Source: CAD feature listing. Evaluate the final solid. Frame: model axes, mm. Round coordinates to 2 decimals unless told otherwise and drop trailing zeros. Order: outer loops, then holes, each group sorted by start corner. A loop starts at its lowest first (then second) coordinate and runs counter-clockwise, first axis right, second up. Notation, with made-up numbers: (-28, 67) - (20, 67) arc R4 ccw to (20, 74) - close; hole circle Ø8 at (21, 44.25). An arc over 180 degrees is marked (long way). Put each result on its own line as item: value. Start each with the question number.
1) Section A-A on y = -0.8. Output: boundary loops of the cut face in (x, z), then the cut area to 3 significant figures.
2) Line query: probe 1 along X at (y, z) = (-1.45, -24); probe 2 along X at (y, z) = (-0.6, -25.5); probe 3 along Z at (x, y) = (-55, 0.1). Output: solid intervals per line, ascending. Write a range as [from, to].
3) Contact query for a flat-ended pin moving along its axis: P1, Ø1.3, axis at y = 1, z = 1, coming from the +X side. Output: stop coordinate, or through.
4) Section B-B on z = 11. Output: boundary loops of the cut face in (x, y).
```python
from build123d import *

# Parameters (mm, degrees)
SKETCH1_R           = 2.2479
BOSS_EXTRUDE1_DEPTH = 1.5875


with BuildPart() as part:
    # Sketch1 → Boss-Extrude1 (new, symmetric)
    with BuildSketch(Plane(origin=(0, 0, 0), x_dir=(1, 0, 0), z_dir=(0, 1, 0))):
        with BuildLine():
            Line((-47.25, 6.976491924), (-47.25, -6.976491924))
            ThreePointArc((-47.25, -6.976491924), (-49.69071054, -13.523028631), (-55.821428571, -16.87392511))
            ThreePointArc((-55.821428571, -16.87392511), (-60.419467095, -19.38709747), (-62.25, -24.297))
            ThreePointArc((-62.25, -24.297), (-60.053300859, -29.600300859), (-54.75, -31.797))
            Line((-54.75, -31.797), (54.75, -31.797))
            ThreePointArc((54.75, -31.797), (60.053300859, -29.600300859), (62.25, -24.297))
            ThreePointArc((62.25, -24.297), (60.419467095, -19.38709747), (55.821428571, -16.87392511))
            ThreePointArc((55.821428571, -16.87392511), (49.69071054, -13.523028631), (47.25, -6.976491924))
            Line((47.25, -6.976491924), (47.25, 6.976491924))
            ThreePointArc((47.25, 6.976491924), (49.69071054, 13.523028631), (55.821428571, 16.87392511))
            ThreePointArc((55.821428571, 16.87392511), (60.419467095, 19.38709747), (62.25, 24.297))
            ThreePointArc((62.25, 24.297), (60.053300859, 29.600300859), (54.75, 31.797))
            Line((54.75, 31.797), (-54.75, 31.797))
            ThreePointArc((-54.75, 31.797), (-60.053300859, 29.600300859), (-62.25, 24.297))
            ThreePointArc((-62.25, 24.297), (-60.419467095, 19.38709747), (-55.821428571, 16.87392511))
            ThreePointArc((-55.821428571, 16.87392511), (-49.69071054, 13.523028631), (-47.25, 6.976491924))
        make_face()
        with Locations(Location((54.75, 24.297, 0), (0, 0, 270))):
            Circle(SKETCH1_R, mode=Mode.SUBTRACT)
        with Locations(Location((54.75, -24.297, 0), (0, 0, 270))):
            Circle(SKETCH1_R, mode=Mode.SUBTRACT)
        with Locations(Location((-54.75, -24.297, 0), (0, 0, 270))):
            Circle(SKETCH1_R, mode=Mode.SUBTRACT)
        with Locations(Location((-54.75, 24.297, 0), (0, 0, 270))):
            Circle(SKETCH1_R, mode=Mode.SUBTRACT)
    extrude(amount=BOSS_EXTRUDE1_DEPTH, both=True)


solid = part.part
```
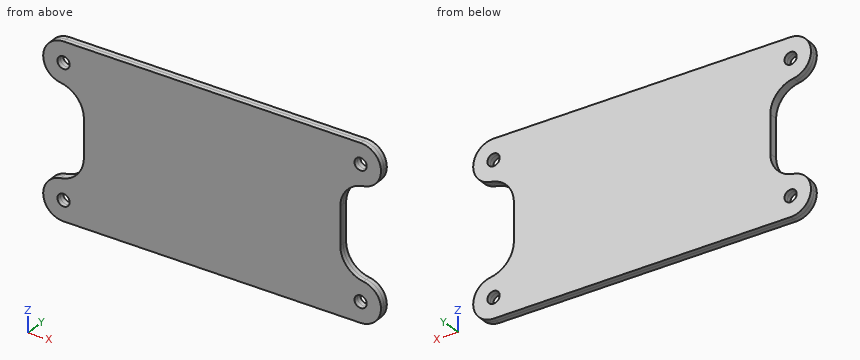
Answer sheet:
1. outline: (-55.82, -16.87) arc R7.5 ccw to (-54.75, -31.8) - (54.75, -31.8) arc R7.5 ccw to (55.82, -16.87) arc R10 cw to (47.25, -6.98) - (47.25, 6.98) arc R10 cw to (55.82, 16.87) arc R7.5 ccw to (54.75, 31.8) - (-54.75, 31.8) arc R7.5 ccw to (-55.82, 16.87) arc R10 cw to (-47.25, 6.98) - (-47.25, -6.98) arc R10 cw to start; hole circle Ø4.5 at (-54.75, -24.3); hole circle Ø4.5 at (-54.75, 24.3); hole circle Ø4.5 at (54.75, -24.3); hole circle Ø4.5 at (54.75, 24.3)
1. area: 6,830 mm^2
2. probe 1: [-62.24, -56.98], [-52.52, 52.52], [56.98, 62.24]
2. probe 2: [-62.15, -56.65], [-52.85, 52.85], [56.65, 62.15]
2. probe 3: [-31.79, -26.53], [-22.06, -16.72], [16.72, 22.06], [26.53, 31.79]
3. P1: x = 47.25
4. outline: (-48.1, -1.59) - (48.1, -1.59) - (48.1, 1.59) - (-48.1, 1.59) - close
